Geometry: final body of the model. Coordinates: model frame, mm. Face numbers are marked on the shaded views. A direction names the side the tool comes from. Round coordinates to 2 decimals unless told otherwise and drop trailing zeros. Loops run counter-clockwise (first coordinate to the right, second up) from the corner with the lowest first, then second, coordinate; pieces in that order, holes last. Notation, with made-up numbers: (30, -20.5) - (57, -20.5) arc R25 ccw to (57, 3.5) - close; hole circle Ø9 at (-23.5, 8.25). An arc over 180 degrees is marked (long way). Return JSON: item names as keys, results as strings. Group by question number.
1. Draft query along X for the marked faces 4, 5 and 6. Return one class per face: +X half, -X half, draft (parallel to the pull), parting line (faces both ways), or undercut.
2. Set-up query: the marked faces 1, 2 and 3. Return all of +Z, -Z, +X, -X, +Y, -Y with unobstructed straight access to the full face (end or side cutting, diameter ignored); none if empty.
3. Section A-A on y = 0. Return loops of the section in (x, z) (3 decimals).
4. Material intervals for probe 1 along X at (y, z) = (6, 1.75); probe 2 along X at (y, z) = (2.75, -2.5); probe 3 along X at (y, z) = (-1, -1.25), sorted ascending.
5. First-contact query: pin 1 Ø10 at (x, z) = (-13.5, 0) entering from +Y; pin 2 Ø2 at (y, z) = (6.5, -2) entering from -X; pin 3 Ø2 at (x, y) = (-8, -2.5) entering from +Z. Flat tips, straight axial feed; report the tip coordinate or a pass-through.
6. Section C-C on x = -6.25. Return loops of the section in (y, z) (3 decimals).
from build123d import *


with BuildPart() as part:
    # Sketch1 → Revolve1 (revolve)
    with BuildSketch(Plane.XY, mode=Mode.PRIVATE) as revolve1_sk:
        Polygon((-22.4892, 1.75), (-8.9892, 1.75), (-8.9892, 6.4963), (-6.9892, 6.4963), (-6.9892, 3.175), (-2.4892, 3.175), (-2.4892, 8.4963), (-1.4892, 8.4963), (0, 3), (0, 1.25), (0.25, 1.25), (0.25, 0), (-22.4892, 0), align=None)
    revolve(revolve1_sk.sketch.rotate(Axis((-22.4892, 0, 0), (-1, 0, 0)), 90), axis=Axis((-22.4892, 0, 0), (-1, 0, 0)))


solid = part.part
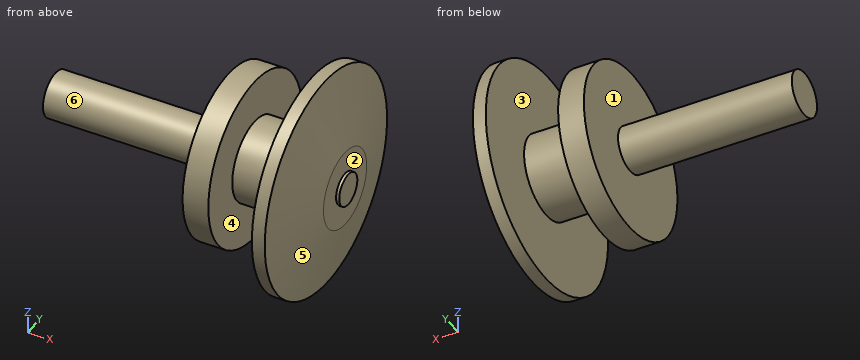
Taken from the geometry:
{
 "1": {"face 4": "undercut", "face 5": "+X half", "face 6": "draft"},
 "2": {"face 1": "-X", "face 2": "+X", "face 3": "none"},
 "3": {"outline": "(-22.489, -1.75) - (-8.989, -1.75) - (-8.989, -6.496) - (-6.989, -6.496) - (-6.989, -3.175) - (-2.489, -3.175) - (-2.489, -8.496) - (-1.489, -8.496) - (0, -3) - (0, -1.25) - (0.25, -1.25) - (0.25, 1.25) - (0, 1.25) - (0, 3) - (-1.489, 8.496) - (-2.489, 8.496) - (-2.489, 3.175) - (-6.989, 3.175) - (-6.989, 6.496) - (-8.989, 6.496) - (-8.989, 1.75) - (-22.489, 1.75) - close"},
 "4": {"probe 1": "-8.99 to -6.99, -2.49 to -0.88", "probe 2": "-8.99 to -6.99, -2.49 to -0.19", "probe 3": "-22.49 to 0"},
 "5": {"pin 1": "y = 6.5", "pin 2": "x = -8.99", "pin 3": "z = 6.32"},
 "6": {"outline": "circle Ø6.35 at (0, 0)"}
}
